Input: part model. Units: mm. Frame: model coordinates. Face numbers are marked on the shaded views. Coordinates: 2 decimals unless noted, no trailing zeros. Loops run counter-clockwise (first coordinate to the right, second up) from the corner with the lowest first, then second, coordinate; pieces in that order, holes last.
Item 1: Contact query for flat-ended pins moving along their axis: P1, Ø3, axis at y = -61, z = -17, coming from the +X side; P2, Ø4, axis at x = 27, y = 31, coming from the +Z side; P3, Ø6, axis at y = -667, z = -24, coming from the +X side. Output: stop coordinate, or through.
Item 2: Section C-C on y = -728. Return loops of the section in (x, z), and give its area (3 significant figures).
Item 3: Section B-B on z = 0. Return loops of the section in (x, y), and give its area (3 significant figures).
Item 4: Section D-D on y = 26. Return loops of the section in (x, z).
Item 5: Section A-A on x = 0. Return loops of the section in (y, z).
Item 6: Ray query, line 1 along Y through (x, z) = (-2, -1.5). Return the intervals inside material, ascending.
Item 7: Pull-direction query (Y, two-part tool) for the marked faces 1, 2 and 3; classes: released by +Y, released by -Y, zero draft, split by the parting line, or undercut.
```python
from build123d import *

# Parameters (mm, degrees)
SKETCH1_R           = 30
EXTRUDE1_DEPTH      = 800
SKETCH_1_R          = 10
CUT_EXTRUDE_1_DEPTH = 35.6


# Read off the part's stored shape, not the designer's step: 连接重组1
with BuildPart() as part:
    # Sketch1 → Extrude1 (new body)
    with BuildSketch(Plane(origin=(0, 0, 0), x_dir=(1, 0, 0), z_dir=(0, 1, 0))):
        with Locations(Location((0, 0, 0), (0, 0, 270))):
            Circle(SKETCH1_R)
    extrude(amount=-EXTRUDE1_DEPTH)

    # 草图1 → 切除-拉伸1 (cut)
    with BuildSketch(Plane(origin=(0, 0, 0), x_dir=(1, 0, 0), z_dir=(0, 1, 0))):
        with Locations(Location((0, 0, 0), (0, 0, 270))):
            Circle(SKETCH_1_R)
    extrude(amount=-CUT_EXTRUDE_1_DEPTH, mode=Mode.SUBTRACT)

    # 连接重组1 outline → 连接重组1 (revolve)
    with BuildSketch(Plane.XY):
        with BuildLine():
            ThreePointArc((22.543988515, 62.888907458), (22.516451416, 64.161768918), (23.262631751, 65.193345138))
            ThreePointArc((23.262631751, 65.193345138), (38.089361999, 109.948085758), (0, 137.73332))
            Line((0, 137.73332), (0, -35.6))
            Line((0, -35.6), (10, -35.6))
            Line((10, -35.6), (10, 0))
            Line((10, 0), (30, 0))
            Line((30, 0), (39.999998202, -3.56e-06))
            Line((39.999998202, -3.56e-06), (39.999998202, 14.399991661))
            Line((39.999998202, 14.399991661), (22.543988515, 62.888907458))
        make_face()
    revolve(axis=Axis((0, 0, 0), (0, 1, 0)))


solid = part.part
```
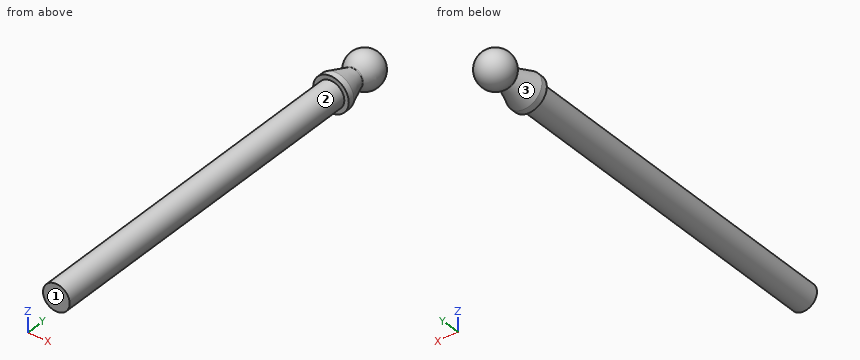
Results found:
1. P1: stops at x = 25.69
1. P2: stops at z = 23.32
1. P3: stops at x = 21.42
2. outline: circle Ø60 at (0, 0)
2. area: 2,830 mm2
3. outline: (-40, 0) - (-30, 0) - (-30, -800) - (30, -800) - (30, 0) - (40, 0) - (40, 14.4) - (22.54, 62.89) arc R2 cw to (23.26, 65.19) arc R40 ccw (long way) to (-23.26, 65.19) arc R2 cw to (-22.54, 62.89) - (-40, 14.4) - close
3. area: 57,100 mm2
4. outline: circle Ø71.65 at (0, 0)
5. outline: (-800, -30) - (0, -30) - (0, -40) - (14.4, -40) - (62.89, -22.54) arc R2 cw to (65.19, -23.26) arc R40 ccw (long way) to (65.19, 23.26) arc R2 cw to (62.89, 22.54) - (14.4, 40) - (0, 40) - (0, 30) - (-800, 30) - close
6. line 1: y = -800 to 137.66
7. face 1: released by -Y
7. face 2: zero draft
7. face 3: undercut
